```python
from build123d import *

# Parameters (mm, degrees)
SKETCH1_R           = 7.25
SKETCH1_R_2         = 6.1
BOSS_EXTRUDE1_DEPTH = 1
SKETCH2_R           = 7.25
SKETCH2_R_2         = 6.1
BOSS_EXTRUDE4_DEPTH = 19
BOSS_EXTRUDE5_START = -2
SKETCH3_W           = 34.5
SKETCH3_H           = 10.25
BOSS_EXTRUDE5_DEPTH = 7
SKETCH4_R           = 0.5
CUT_EXTRUDE1_DEPTH  = 10


with BuildPart() as part:
    # Sketch1 → Boss-Extrude1 (new, symmetric)
    # profile 1 of 2: a face of its own
    with BuildSketch(Plane.XY):
        with BuildLine():
            Line((11.5, -16), (11.5, -5.505678886))
            ThreePointArc((11.5, -5.505678886), (12.75, 0), (11.5, 5.505678886))
            Line((11.5, 5.505678886), (11.5, 16))
            Line((11.5, 16), (-11.5, 16))
            Line((-11.5, 16), (-11.5, 5.505678886))
            ThreePointArc((-11.5, 5.505678886), (-12.75, 0), (-11.5, -5.505678886))
            Line((-11.5, -5.505678886), (-11.5, -16))
            Line((-11.5, -16), (11.5, -16))
        make_face()
        Circle(SKETCH1_R, mode=Mode.SUBTRACT)
    # profile 2 of 2: a face of its own
    with BuildSketch(Plane.XY):
        Circle(SKETCH1_R)
        Circle(SKETCH1_R_2, mode=Mode.SUBTRACT)
    boss_extrude1 = extrude(amount=BOSS_EXTRUDE1_DEPTH, both=True)

    # Sketch2 → Boss-Extrude4 (add)
    with BuildSketch(Plane.XY.offset(1)):
        Circle(SKETCH2_R)
        Circle(SKETCH2_R_2, mode=Mode.SUBTRACT)
    extrude(amount=BOSS_EXTRUDE4_DEPTH)

    # Sketch3 → Boss-Extrude5 (add)
    with BuildSketch(Plane(origin=(0, 0, -1), x_dir=(-1, 0, 0), z_dir=(0, 0, -1)).offset(BOSS_EXTRUDE5_START)):
        with Locations((0, 10.875)):
            Rectangle(SKETCH3_W, SKETCH3_H)
        with Locations((0, -10.875)):
            Rectangle(SKETCH3_W, SKETCH3_H)
    boss_extrude5 = extrude(amount=BOSS_EXTRUDE5_DEPTH)

    # Mirror1: Boss-Extrude1, Boss-Extrude5 across plane
    add(boss_extrude1.mirror(Plane.XY.offset(10.5)))
    add(boss_extrude5.mirror(Plane.XY.offset(10.5)))

    # Sketch4 → Cut-Extrude1 (cut)
    with BuildSketch(Plane(origin=(0, 0, -6), x_dir=(-1, 0, 0), z_dir=(0, 0, -1))):
        with Locations((-11.5, 14)):
            Circle(SKETCH4_R)
        with Locations((-3.75, 14)):
            Circle(SKETCH4_R)
        with Locations(Location((3.75, 14, 0), (0, 0, 180))):
            Circle(SKETCH4_R)
        with Locations(Location((11.5, 14, 0), (0, 0, 180))):
            Circle(SKETCH4_R)
        with Locations((3.75, -14)):
            Circle(SKETCH4_R)
        with Locations(Location((-3.75, -14, 0), (0, 0, 180))):
            Circle(SKETCH4_R)
        with Locations(Location((-11.5, -14, 0), (0, 0, 180))):
            Circle(SKETCH4_R)
        with Locations((11.5, -14)):
            Circle(SKETCH4_R)
    extrude(amount=-CUT_EXTRUDE1_DEPTH, mode=Mode.SUBTRACT)


solid = part.part
```
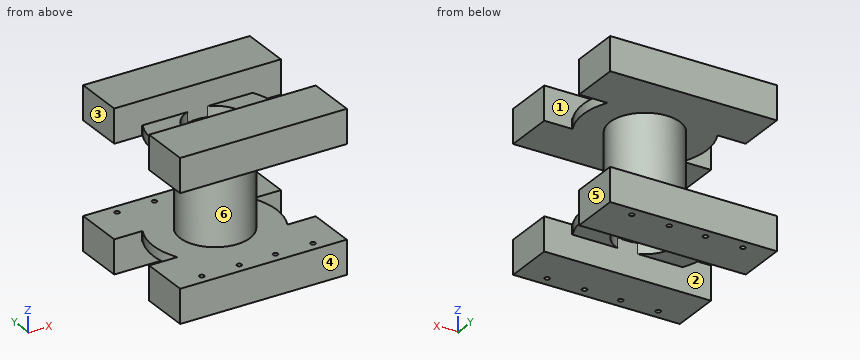
CAD build for the part. Positions are in the model's coordinates, mm. Face numbers are marked on the shaded views. A direction names the side the tool comes from. Round coordinates to 2 decimals unless told otherwise and drop trailing zeros. Loops run counter-clockwise (first coordinate to the right, second up) from the corner with the lowest first, then second, coordinate; pieces in that order, holes last. Notation, with made-up numbers: (-35, -35) - (-4, -35) arc R20 cw to (-4, -25) - close; hole circle Ø5 at (60.25, 77). An arc over 180 degrees is marked (long way). Return JSON: item names as keys, results as strings. Group by question number.
Q1. Band-saw the part on D-D on y = 14. Give the cut face in (x, z), plus the area to 3 significant figures.
Q2. Drill centre lines: line 1 along Y through (x, z) = (11.5, -2.75); line 2 along Z through (x, y) = (7.5, 14); line 3 along Y through (x, z) = (15, -1.5). Where is each one in solid material? Low to high. Write a range as [from, to].
Q3. Band-saw the part on A-A on y = 0. Give the cut face in (x, z), plus the area to 3 significant figures.
Q4. Band-saw the part on B-B on z = 24. Give the cut face in (x, y), plus the area to 3 significant figures.
Q5. Two-plate mould, pull along Y, no slides. Class the marked faces 1, 2, 3 and 4: +Y half, -Y half, draft (parallel to the pull), parting line (faces both ways), or undercut.
Q6. Tool access for the marked faces 5 and 6: list every direction of +Z, -Z, +X, -X, +Y, -Y with a clear straight run to the whole face (end or side of a thin tool).
Q7. Band-saw the part on C-C on x = 0. Give the cut face in (y, z), plus the area to 3 significant figures.
Q8. Flat gauge pins, fed straight in: pin 1 Ø5.5 at (x, y) = (6.5, -2) entering from +Z; pin 2 Ø1.5 at (y, z) = (5, 19.5) entering from -X; pin 3 Ø2 at (x, z) = (-0.5, 13.5) entering from -Y. Where does each tip first touch, or does it go through?
Solutions:
{
 "1": {"outline": "(-17.25, -6) - (-12, -6) - (-12, 1) - (-17.25, 1) - close; (-17.25, 20) - (17.25, 20) - (17.25, 27) - (-17.25, 27) - close; (-11, -6) - (-4.25, -6) - (-4.25, 1) - (-11, 1) - close; (-3.25, -6) - (3.25, -6) - (3.25, 1) - (-3.25, 1) - close; (4.25, -6) - (11, -6) - (11, 1) - (4.25, 1) - close; (12, -6) - (17.25, -6) - (17.25, 1) - (12, 1) - close", "area": "455 mm^2"},
 "2": {"line 1": "y = [-16, -14.5], [-13.5, -5.75], [5.75, 13.5], [14.5, 16]", "line 2": "z = [-6, 1], [20, 27]", "line 3": "y = [-16, -5.75], [5.75, 16]"},
 "3": {"outline": "(-12.75, -1) - (-6.1, -1) - (-6.1, 22) - (-12.75, 22) - (-12.75, 20) - (-7.25, 20) - (-7.25, 1) - (-12.75, 1) - close; (6.1, -1) - (12.75, -1) - (12.75, 1) - (7.25, 1) - (7.25, 20) - (12.75, 20) - (12.75, 22) - (6.1, 22) - close", "area": "96.9 mm^2"},
 "4": {"outline": "(-17.25, -16) - (17.25, -16) - (17.25, -5.75) - (-17.25, -5.75) - close; (-17.25, 5.75) - (17.25, 5.75) - (17.25, 16) - (-17.25, 16) - close", "area": "707 mm^2"},
 "5": {"face 1": "undercut", "face 2": "undercut", "face 3": "draft", "face 4": "-Y half"},
 "6": {"face 5": "+Z, -Z, +X, +Y, -Y", "face 6": "none"},
 "7": {"outline": "(-16, -6) - (-5.75, -6) - (-5.75, 1) - (-6.1, 1) - (-6.1, 20) - (-5.75, 20) - (-5.75, 27) - (-16, 27) - (-16, 20) - (-7.25, 20) - (-7.25, 1) - (-16, 1) - close; (5.75, -6) - (16, -6) - (16, 1) - (7.25, 1) - (7.25, 20) - (16, 20) - (16, 27) - (5.75, 27) - (5.75, 20) - (6.1, 20) - (6.1, 1) - (5.75, 1) - close", "area": "331 mm^2"},
 "8": {"pin 1": "stops at z = 22", "pin 2": "stops at x = -11.95", "pin 3": "stops at y = -7.25"}
}
